from build123d import *

# Parameters (mm, degrees)
F0_W     = 7.62
F0_H     = 48.07742
F1_DEPTH = 127
F0_H_2   = 66.986127
F2_DEPTH = 127
F3_DEPTH = 114.3
F0_H_3   = 25.906453
F4_DEPTH = 127


with BuildPart() as f1:
    # F0 (on Top) → F1 (new body)
    with BuildSketch(Plane.XY):
        Polygon((121.709297, 79.080492), (-111.970703, 79.080492), (-111.970703, 71.460492), (114.089297, 71.460492), (121.709297, 71.460492), align=None)
        with Locations((117.899297, 47.421782)):
            Rectangle(F0_W, F0_H)
    extrude(amount=F1_DEPTH)

    # F0 (on Top) → F2 (join)
    with BuildSketch(Plane.XY):
        with Locations((117.899297, -10.109991)):
            Rectangle(F0_W, F0_H_2)
    extrude(amount=F2_DEPTH)

    # F0 (on Top) → F3 (cut)
    with BuildSketch(Plane.XY):
        with Locations((117.899297, -10.109991)):
            Rectangle(F0_W, F0_H_2)
    extrude(amount=F3_DEPTH, mode=Mode.SUBTRACT)

    # F0 (on Top) → F4 (join)
    with BuildSketch(Plane.XY):
        with Locations((117.899297, -56.556281)):
            Rectangle(F0_W, F0_H_3)
    extrude(amount=F4_DEPTH)


solid = f1.part
Here's how the part is built. I have some questions about the finished solid (model axes, mm). A direction names the side the tool comes from. Round coordinates to 2 decimals unless told otherwise and drop trailing zeros. Order: outer loops, then holes, each group sorted by start corner. A loop starts at its lowest first (then second) coordinate and runs counter-clockwise, first axis right, second up. Notation, with made-up numbers: (-36, 5.25) -> (8, 5.25) arc R19 ccw to (8, 26.25) -> close; hole circle Ø2 at (-32.5, 14). An arc over 180 degrees is marked (long way). Return JSON: item names as keys, results as strings.
Q1. If we section it at C-C on x = -81.5: List the corners of the cut face in (y, z) for me, plus the area to 3 significant figures.
Filled sheet:
{"outline": "(71.46, 0) -> (79.08, 0) -> (79.08, 127) -> (71.46, 127) -> close", "area": "968 mm^2"}
Q2. Which directions (+Z, -Z, +X, -X, +Y, -Y) give clear straight access to the entire face, cutting with the end or side of a thin tool? Please do faces 1 (the flat face through (118, 23.383, 56)), 2 (the flat face through (-111.971, 75, 63)), 3 (the flat face through (114.089, 31, 63)).
Filled sheet:
{"face 1": "-Z, +X, -X", "face 2": "+Z, -Z, -X, +Y, -Y", "face 3": "+Z, -Z, -X, -Y"}
Q3. I need wall thicknesses on line 1 along Y through (x, z) = (-31.5, 17); line 2 along X through (y, z) = (45, 89). Which ranges of each line are inside material? Lowest first, please. Write a range as from..to.
Filled sheet:
{"line 1": "y = 71.46..79.08", "line 2": "x = 114.09..121.71"}
Q4. For pin 1 Ø5 at (x, z) = (-58.5, 71.5) entering from -Y; pin 2 Ø3 at (y, z) = (43.5, 19) entering from -X; pin 3 Ø2.5 at (x, y) = (116.5, -18.5) entering from -Z, each with a flat end and sliding along its axis, tell me the tip position at first contact or that it passes through.
Filled sheet:
{"pin 1": "stops at y = 71.46", "pin 2": "stops at x = 114.09", "pin 3": "stops at z = 114.3"}
Q5. If we mould it in two halves opening along Y, with no side actions, what happens to faces 4 (the flat face through (118, -69.51, 63)), 5 (the flat face through (118, -56, 0)), 6 (the flat face through (118, -10, 114.3))? For each: released by +Y, released by -Y, zero draft, split by the parting line, or undercut.
Filled sheet:
{"face 4": "released by -Y", "face 5": "zero draft", "face 6": "undercut"}
Q6. If we section it at B-B on y = -37.5: List the corners of the cut face in (x, z) for me.
Filled sheet:
{"outline": "(114.09, 114.3) -> (121.71, 114.3) -> (121.71, 127) -> (114.09, 127) -> close"}
Q7. If we section it at A-A on z = 77.5: List the corners of the cut face in (x, y) for me.
Filled sheet:
{"outline": "(-111.97, 71.46) -> (114.09, 71.46) -> (114.09, 23.38) -> (121.71, 23.38) -> (121.71, 79.08) -> (-111.97, 79.08) -> close; (114.09, -69.51) -> (121.71, -69.51) -> (121.71, -43.6) -> (114.09, -43.6) -> close"}
